Could you check a few things on this drawing? It's one solid part, dimensions in mm from its lowest x, y, z. Round coordinates to 2 decimals unless told otherwise and drop trailing zeros. Loops run counter-clockwise (first coordinate to the right, second up) from the corner with the lowest first, then second, coordinate; pieces in that order, holes last. Notation, with made-up numbers: (30.25, 88) -> (69.25, 88) arc R21 ccw to (69.25, 125) -> close; hole circle Ø9 at (37.25, -1). An arc over 180 degrees is marked (long way). Use one line per item in the form item = value. Start each with the question number.
Item 1: If we section it at C-C (x = 23.5): Write out the boundary of the cut face in (y, z).
Item 2: If we section it at A-A (z = 133): Write out the boundary of the cut face in (x, y).
Item 3: If we section it at B-B (y = 1.8): Write out the boundary of the cut face in (x, z).
Item 4: I'm going to push flat-ended pins straight in: pin 1 Ø1.5 at (y, z) = (0.5, 126) entering from +X; pin 2 Ø0.9 at (x, y) = (28, 1) entering from +Z; pin 3 Ø0.9 at (x, y) = (5.5, 2) entering from -Z. Where does each tip first touch, or does it pass through?
Item 5: If I drill on L1, parallel to X at y = 0.8, z = 166; L2, parallel to Z at x = 47.5, y = 2.5, over which ranges is the centre line in solid material (lowest first)? Write a range as [from, to].
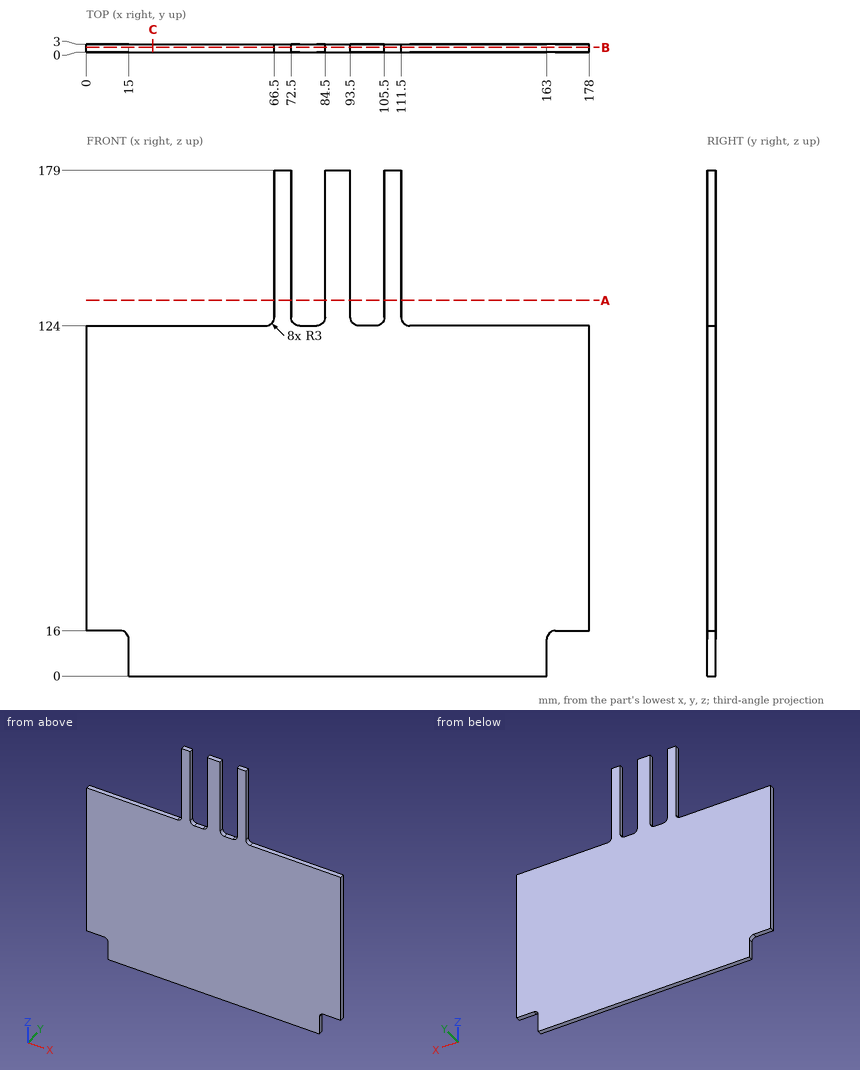
Values found:
q1.outline = (0, 0) -> (3, 0) -> (3, 124) -> (0, 124) -> close
q2.outline = (66.5, 0) -> (72.5, 0) -> (72.5, 3) -> (66.5, 3) -> close; (84.5, 0) -> (93.5, 0) -> (93.5, 3) -> (84.5, 3) -> close; (105.5, 0) -> (111.5, 0) -> (111.5, 3) -> (105.5, 3) -> close
q3.outline = (0, 16) -> (12, 16) arc R3 cw to (15, 13) -> (15, 0) -> (163, 0) -> (163, 13) arc R3 cw to (166, 16) -> (178, 16) -> (178, 124) -> (114.5, 124) arc R3 cw to (111.5, 127) -> (111.5, 179) -> (105.5, 179) -> (105.5, 127) arc R3 cw to (102.5, 124) -> (96.5, 124) arc R3 cw to (93.5, 127) -> (93.5, 179) -> (84.5, 179) -> (84.5, 127) arc R3 cw to (81.5, 124) -> (75.5, 124) arc R3 cw to (72.5, 127) -> (72.5, 179) -> (66.5, 179) -> (66.5, 127) arc R3 cw to (63.5, 124) -> (0, 124) -> close
q4.pin_1 = 112.06
q4.pin_2 = 124
q4.pin_3 = 16
q5.L1 = [66.5, 72.5], [84.5, 93.5], [105.5, 111.5]
q5.L2 = [0, 124]
